Design review of the part shown in the three views and the two pictorial views. Dimensions are in mm from the part's minimum x, y and z. A direction names the side the tool comes from. Give positions to 0.01 mm unless a question says otherwise; leave off trailing zeros. Order: outer loops, then holes, each group sorted by start corner. A loop starts at its lowest first (then second) coordinate and runs counter-clockwise, first axis right, second up.
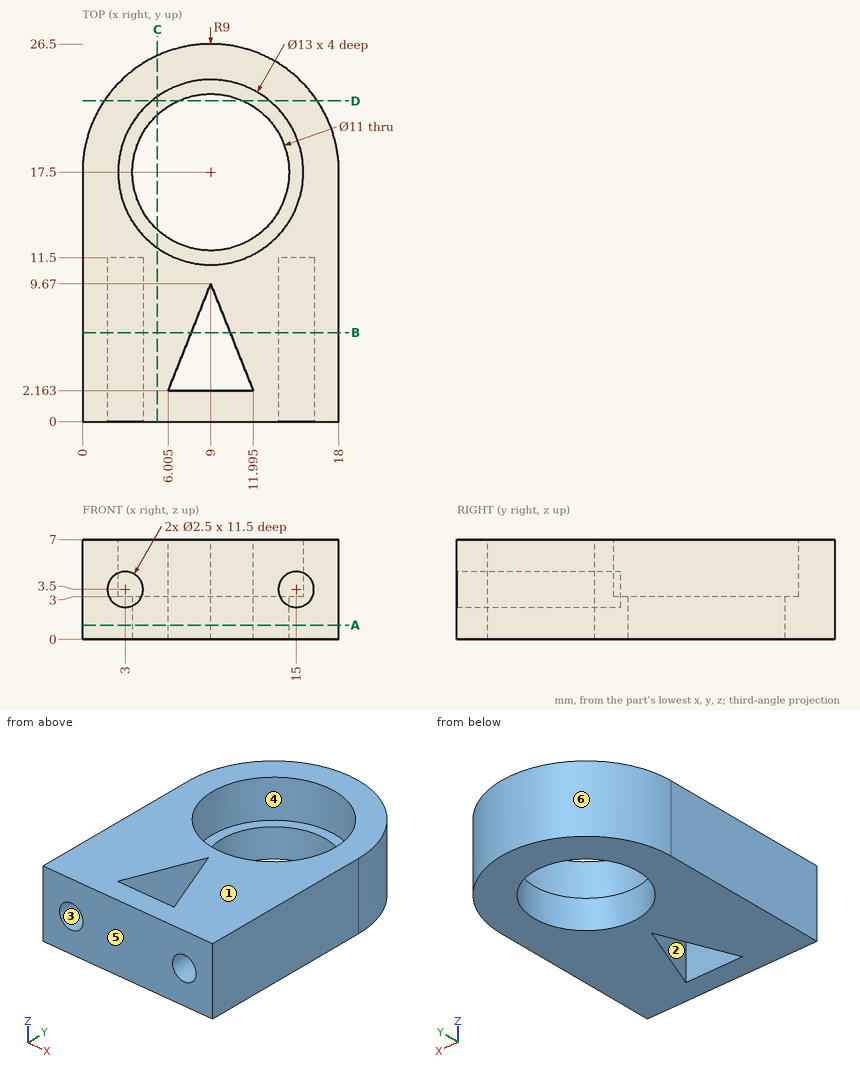
Item 1: Draft analysis for pull direction X (two halves, no side actions). For the marked faces 4, 5 and 6, state which applies: released by +X, released by -X, zero draft, split by the parting line, or undercut.
Values found:
face 4: undercut
face 5: zero draft
face 6: split by the parting line
Item 2: Clearance check with flat-ended pins moving along their axes: pin 1 Ø2 at (x, z) = (3, 3.5) entering from +Y; pin 2 Ø4 at (y, z) = (23, 6) entering from -X; pin 3 Ø8 at (x, y) = (9, 17.5) entering from -Z; pin 4 Ø1.5 at (x, z) = (5.5, 1) entering from +Y. State where each tip first meets the part, or that it passes through.
Values found:
pin 1: stops at y = 24.98
pin 2: stops at x = 0.71
pin 3: passes through
pin 4: stops at y = 26.07
Item 3: For line 1 (X direction, y = 17.5, z = 1.3); line 2 (X direction, y = 4.75, z = 3.5); line 3 (X direction, y = 16, z = 2), list the stretches that pass through material, from the lowest coordinate up.
Values found:
line 1: x = 0 to 3.5, 14.5 to 18
line 2: x = 0 to 1.75, 4.25 to 7.04, 10.96 to 13.75, 16.25 to 18
line 3: x = 0 to 3.71, 14.29 to 18
Item 4: Take a section at D-D (y = 22.5). Give the boundary of the cut face in (x, z).
Values found:
outline: (1.52, 0) - (6.71, 0) - (6.71, 3) - (4.85, 3) - (4.85, 7) - (1.52, 7) - close; (11.29, 0) - (16.48, 0) - (16.48, 7) - (13.15, 7) - (13.15, 3) - (11.29, 3) - close
Item 5: Take a section at C-C (x = 5.25). Give the boundary of the cut face in (y, z), and give its area (3 significant figures).
Values found:
outline: (0, 0) - (13.48, 0) - (13.48, 3) - (12.19, 3) - (12.19, 7) - (0, 7) - close; (21.52, 0) - (25.68, 0) - (25.68, 7) - (22.81, 7) - (22.81, 3) - (21.52, 3) - close
area: 113 mm2
Item 6: Take a section at A-A (z = 1). Give the boundary of the cut face in (x, y) (1 decimal).
Values found:
outline: (0, 0) - (18, 0) - (18, 17.5) arc R9 ccw to (0, 17.5) - close; hole circle Ø11 at (9, 17.5); hole (6, 2.2) - (12, 2.2) - (9, 9.7) - close
Item 7: Take a section at B-B (y = 6.25). Give the number of separate pieces and of enclosed holes in the cut face.
Values found:
separate pieces: 2
enclosed holes: 2
Item 8: For the marked faces 1, 2 and 3, list the 3-axis set-ups (+Z, -Z, +X, -X, +Y, -Y) from which the entire face can be reached by the end or side of a thin tool; tool diameter is ignored.
Values found:
face 1: +Z, +X, -X, +Y, -Y
face 2: +Z, -Z
face 3: -Y
